Source: CAD feature listing. Evaluate the final solid. Frame: model axes, mm. Face numbers are marked on the shaded views. A direction names the side the tool comes from. Give positions to 0.01 mm unless a question says otherwise; leave off trailing zeros. Write each loop counter-clockwise with the first axis right and the second up, starting at its lowest first coordinate (ties: lowest second). Pieces come first, ordered by that corner, then holes. Notation, with made-up numbers: (18, 29) -> (44, 29) arc R17 cw to (44, 39) -> close; hole circle Ø9 at (-39.75, -18.75). An arc over 180 degrees is marked (long way). Answer as a JSON object with one key per item and string values. Group by question number.
Item 1: First-contact query: pin 1 Ø3.5 at (x, y) = (-2, -10) entering from +Z; pin 2 Ø4 at (x, z) = (0.5, -5.5) entering from +Y; pin 3 Ø1.5 at (x, y) = (-2, -2) entering from +Z; pin 4 Ø3.5 at (x, y) = (-0.5, -137) entering from -Z. Flat tips, straight axial feed; report the tip coordinate or a pass-through.
Item 2: Section query B-B on x = 2.25. Return the cut outline in (y, z), plus the area to 3 significant figures.
Item 3: Pull-direction query (X, two-part tool) for the marked faces 5, 6 and 7; classes: pulls with the +X half, pulls with the -X half, needs draft (parallel to the pull), parting line crosses it, or undercut.
Item 4: Ray query, probe 1 along Y at (x, z) = (-4.5, -6); probe 2 along X at (y, z) = (-10, -7.25); probe 3 along Y at (x, z) = (6.5, -4.75). Return the intervals inside material, ascending. Write a range as from..to.
Item 5: Access query for the marked faces 1, 2, 3 and 4. Directions: +Z, -Z, +X, -X, +Y, -Y. A direction counts if a zero-diameter tool reaches every point of the face in a straight line with its end or side. Return the directions, or none.
Item 6: Section query C-C on z = 3.5. Return the cut outline in (x, y), plus the area to 3 significant figures.
Item 7: Section query A-A on z = -4.5. Return the cut outline in (x, y), plus the area to 3 significant figures.
from build123d import *

# Parameters (mm, degrees)
F0_W     = 18
F0_H     = 25
F1_DEPTH = 150
F3_DEPTH = 25
F4_W     = 3
F4_H     = 15
F5_DEPTH = 25
F6_W     = 12
F6_H     = 12
F7_DEPTH = 20
F8_W     = 12
F8_H     = 15
F9_DEPTH = 5


with BuildPart() as f1:
    # F0 (on Front) → F1 (new body)
    with BuildSketch(Plane.XZ):
        Rectangle(F0_W, F0_H)
    extrude(amount=F1_DEPTH)

    # F2 (on face) → F3 (cut)
    with BuildSketch(Plane.YZ.offset(9)):
        Polygon((-150, -12.5), (-135, -12.5), (-135, -2.5), (-138, -2.5), (-138, -7.5), (-150, -7.5), align=None)
    extrude(amount=-F3_DEPTH, mode=Mode.SUBTRACT)

    # F4 (on face) → F5 (cut)
    with BuildSketch(Plane.XY.offset(12.5)):
        with Locations((7.5, -142.5)):
            Rectangle(F4_W, F4_H)
        with Locations((-7.5, -142.5)):
            Rectangle(F4_W, F4_H)
    extrude(amount=-F5_DEPTH, mode=Mode.SUBTRACT)

    # F6 (on face) → F7 (cut)
    with BuildSketch(Plane.XY.offset(12.5)):
        with Locations((0, -9)):
            Rectangle(F6_W, F6_H)
    extrude(amount=-F7_DEPTH, mode=Mode.SUBTRACT)

    # F8 (on face) → F9 (cut)
    with BuildSketch(Plane.XZ):
        with Locations((0, 5.012322)):
            Rectangle(F8_W, F8_H)
    extrude(amount=F9_DEPTH, mode=Mode.SUBTRACT)


solid = f1.part
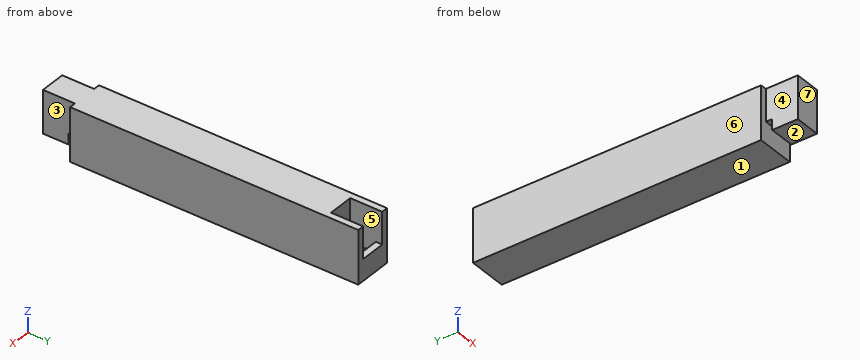
Worked answers:
{
 "1": {"pin 1": "z = -7.5", "pin 2": "y = 0", "pin 3": "z = -2.49", "pin 4": "z = -7.5"},
 "2": {"outline": "(-150, -7.5) -> (-138, -7.5) -> (-138, -2.5) -> (-135, -2.5) -> (-135, -12.5) -> (0, -12.5) -> (0, -2.49) -> (-3, -2.49) -> (-3, -7.5) -> (-15, -7.5) -> (-15, 12.5) -> (-150, 12.5) -> close", "area": "3,380 mm^2"},
 "3": {"face 5": "undercut", "face 6": "pulls with the -X half", "face 7": "needs draft"},
 "4": {"probe 1": "-150..-138, -135..-15, -3..0", "probe 2": "-9..-6, 6..9", "probe 3": "-135..0"},
 "5": {"face 1": "-Z, +X, -X, +Y, -Y", "face 2": "-Z, +X, -X, -Y", "face 3": "+Z, -Z, +X, -Y", "face 4": "+Z, -Z, -X, -Y"},
 "6": {"outline": "(-9, -135) -> (-6, -135) -> (-6, -150) -> (6, -150) -> (6, -135) -> (9, -135) -> (9, 0) -> (6, 0) -> (6, -15) -> (-6, -15) -> (-6, 0) -> (-9, 0) -> close", "area": "2,430 mm^2"},
 "7": {"outline": "(-9, -135) -> (9, -135) -> (9, 0) -> (-9, 0) -> close; (-6, -150) -> (6, -150) -> (6, -138) -> (-6, -138) -> close; hole (-6, -15) -> (6, -15) -> (6, -3) -> (-6, -3) -> close", "area": "2,430 mm^2"}
}
